Design review of the part built by this model. Coordinates are the model's own, in mm. Face numbers are marked on the shaded views. A direction names the side the tool comes from. Coordinates: 2 decimals unless noted, no trailing zeros. Loops run counter-clockwise (first coordinate to the right, second up) from the corner with the lowest first, then second, coordinate; pieces in that order, holes last. Notation, with made-up numbers: (-35, 23.5) -> (16, 23.5) arc R15 ccw to (16, 50.5) -> close; hole circle Ø9 at (28.25, 69.5). An arc over 180 degrees is marked (long way). Use one line per item in the form item = value. Start each with the question number.
1. Consider section A-A (x = 30). State the section outline as (y, z) points, then the cut area to 3 significant figures.
2. Consider section D-D (x = 72). State the section outline as (y, z) points, then the cut area to 3 significant figures.
3. Wall thickness on line 1 (Z direction, x = 50, y = -0.25); line 2 (X direction, y = 2, z = 66.5); line 3 (Z direction, x = 34, y = -1.75): over which ranges is each line inside the solid? List them lowest first. Write a range as from..to.
4. The part is to be moulded in two halves that separate along X. For the marked faces 1, 2, 3 and 4, say which applies: released by +X, released by -X, zero draft, split by the parting line, or undercut.
5. Machinability: for the marked faces 5 and 6, which of the approach directions +Z, -Z, +X, -X, +Y, -Y give a long, thin tool a straight path to every point of the face, cutting with its end or side? Answer none if there is none.
6. Consider section B-B (z = 65). State the section outline as (x, y) points.
7. For pin 1 (5 mm diameter, centred on y = 0, z = 63, fed in from +X); pin 2 (5 mm diameter, centred on x = 6.5, y = -1, fed in from +Z); pin 3 (9.5 mm diameter, centred on x = 50, z = 15, fed in from -Y), all flat-tipped, find the tip position at first contact; note any pin that passes through.
8. Consider section C-C (y = 3). State the section outline as (x, z) points, then the cut area to 3 significant figures.
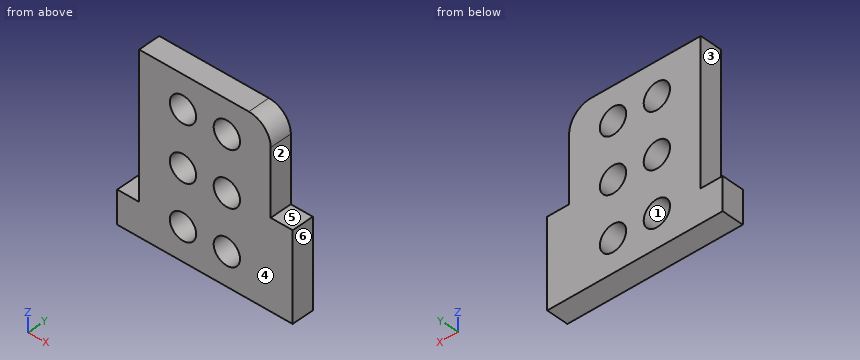
from build123d import *

# Parameters (mm, degrees)
F0_R     = 6
F1_DEPTH = 5


with BuildPart() as f1:
    # F0 (on Front) → F1 (new body, symmetric)
    with BuildSketch(Plane.XZ):
        with BuildLine():
            Line((0, 15), (0, 0))
            Line((0, 0), (80, 0))
            Line((80, 0), (80, 40))
            Line((80, 40), (70, 40))
            Line((70, 40), (70, 70))
            ThreePointArc((70, 70), (67.071068, 77.071068), (60, 80))
            Line((60, 80), (10, 80))
            Line((10, 80), (10, 15))
            Line((10, 15), (0, 15))
        make_face()
        with Locations((30, 15)):
            Circle(F0_R, mode=Mode.SUBTRACT)
        with Locations((50, 15)):
            Circle(F0_R, mode=Mode.SUBTRACT)
        with Locations((30, 40)):
            Circle(F0_R, mode=Mode.SUBTRACT)
        with Locations((30, 65)):
            Circle(F0_R, mode=Mode.SUBTRACT)
        with Locations((50, 40)):
            Circle(F0_R, mode=Mode.SUBTRACT)
        with Locations((50, 65)):
            Circle(F0_R, mode=Mode.SUBTRACT)
    extrude(amount=F1_DEPTH, both=True)


solid = f1.part
Geometry check:
q1.outline = (-5, 0) -> (5, 0) -> (5, 9) -> (-5, 9) -> close; (-5, 21) -> (5, 21) -> (5, 34) -> (-5, 34) -> close; (-5, 46) -> (5, 46) -> (5, 59) -> (-5, 59) -> close; (-5, 71) -> (5, 71) -> (5, 80) -> (-5, 80) -> close
q1.area = 440 mm²
q2.outline = (-5, 0) -> (5, 0) -> (5, 40) -> (-5, 40) -> close
q2.area = 400 mm²
q3.line_1 = 0..9, 21..34, 46..59, 71..80
q3.line_2 = 10..24.19, 35.81..44.19, 55.81..70
q3.line_3 = 0..10.53, 19.47..35.53, 44.47..60.53, 69.47..80
q4.face_1 = undercut
q4.face_2 = released by +X
q4.face_3 = released by -X
q4.face_4 = zero draft
q5.face_5 = +Z, +X, +Y, -Y
q5.face_6 = +Z, -Z, +X, +Y, -Y
q6.outline = (10, -5) -> (24, -5) -> (24, 5) -> (10, 5) -> close; (36, -5) -> (44, -5) -> (44, 5) -> (36, 5) -> close; (56, -5) -> (70, -5) -> (70, 5) -> (56, 5) -> close
q7.pin_1 = 70
q7.pin_2 = 15
q7.pin_3 = through
q8.outline = (0, 0) -> (80, 0) -> (80, 40) -> (70, 40) -> (70, 70) arc R10 ccw to (60, 80) -> (10, 80) -> (10, 15) -> (0, 15) -> close; hole circle Ø12 at (30, 15); hole circle Ø12 at (30, 40); hole circle Ø12 at (30, 65); hole circle Ø12 at (50, 15); hole circle Ø12 at (50, 40); hole circle Ø12 at (50, 65)
q8.area = 4,650 mm²
